```python
from build123d import *

# Parameters (mm, degrees)
SKETCH1_W                 = 100
SKETCH1_H                 = 100
BOSS_EXTRUDE1_DEPTH       = 52
SKETCH2_W                 = 95.5
SKETCH2_H                 = 95.5
BOSS_EXTRUDE2_DEPTH       = 2.5
SKETCH3_W                 = 96
SKETCH3_H                 = 96
CUT_EXTRUDE1_DEPTH        = 13
SKETCH4_R                 = 7.5
CUT_EXTRUDE2_DEPTH        = 37.5
LPATTERN1_COUNT           = 5
LPATTERN1_PITCH           = 17
LPATTERN1_COUNT_DIR2      = 3
LPATTERN1_PITCH_DIR2      = 30
SKETCH_PATTERN1_START     = 17
SKETCH_PATTERN1_OUTLINE_R = 7.5
SKETCH_PATTERN1_DEPTH     = 37.5
FILLET1_R                 = 5
FILLET2_R                 = 2


# Read off the part's stored shape, not the designer's step: Sketch-Pattern1
with BuildPart() as part:
    # Sketch1 → Boss-Extrude1 (new body)
    with BuildSketch(Plane.XY):
        Rectangle(SKETCH1_W, SKETCH1_H)
    extrude(amount=BOSS_EXTRUDE1_DEPTH)

    # Sketch2 → Boss-Extrude2 (add)
    with BuildSketch(Plane.XY.offset(52)):
        Rectangle(SKETCH2_W, SKETCH2_H)
    extrude(amount=BOSS_EXTRUDE2_DEPTH)

    # Sketch3 → Cut-Extrude1 (cut)
    with BuildSketch(Plane(origin=(0, 0, 0), x_dir=(-1, 0, 0), z_dir=(0, 0, -1))):
        Rectangle(SKETCH3_W, SKETCH3_H)
    extrude(amount=-CUT_EXTRUDE1_DEPTH, mode=Mode.SUBTRACT)

    # Sketch4 → Cut-Extrude2 (cut)
    with BuildSketch(Plane.XY.offset(54.5)):
        with Locations((38.75, 38.75)):
            Circle(SKETCH4_R)
    cut_extrude2 = extrude(amount=-CUT_EXTRUDE2_DEPTH, mode=Mode.SUBTRACT)

    # LPattern1: Cut-Extrude2 5 × 3
    with Locations(*[(-j * LPATTERN1_PITCH_DIR2, -i * LPATTERN1_PITCH, 0) for i in range(LPATTERN1_COUNT) for j in range(LPATTERN1_COUNT_DIR2) if (i, j) != (0, 0)]):
        add(cut_extrude2, mode=Mode.SUBTRACT)

    # Sketch-Pattern1 outline → Sketch-Pattern1 (cut)
    with BuildSketch(Plane.XY.offset(SKETCH_PATTERN1_START)):
        with Locations((23.75, 30.5)):
            Circle(SKETCH_PATTERN1_OUTLINE_R)
        with Locations((-36.25, 13.5)):
            Circle(SKETCH_PATTERN1_OUTLINE_R)
        with Locations((23.75, -3.5)):
            Circle(SKETCH_PATTERN1_OUTLINE_R)
        with Locations((-6.25, -3.5)):
            Circle(SKETCH_PATTERN1_OUTLINE_R)
        with Locations((-36.25, -3.5)):
            Circle(SKETCH_PATTERN1_OUTLINE_R)
        with Locations((-6.25, 13.5)):
            Circle(SKETCH_PATTERN1_OUTLINE_R)
        with Locations((23.75, 13.5)):
            Circle(SKETCH_PATTERN1_OUTLINE_R)
        with Locations((-36.25, 30.5)):
            Circle(SKETCH_PATTERN1_OUTLINE_R)
        with Locations((-6.25, 30.5)):
            Circle(SKETCH_PATTERN1_OUTLINE_R)
        with Locations((-36.25, -37.5)):
            Circle(SKETCH_PATTERN1_OUTLINE_R)
        with Locations((-6.25, -37.5)):
            Circle(SKETCH_PATTERN1_OUTLINE_R)
        with Locations((23.75, -20.5)):
            Circle(SKETCH_PATTERN1_OUTLINE_R)
        with Locations((-6.25, -20.5)):
            Circle(SKETCH_PATTERN1_OUTLINE_R)
        with Locations((-36.25, -20.5)):
            Circle(SKETCH_PATTERN1_OUTLINE_R)
        with Locations((23.75, -37.5)):
            Circle(SKETCH_PATTERN1_OUTLINE_R)
    extrude(amount=SKETCH_PATTERN1_DEPTH, mode=Mode.SUBTRACT)

    # Fillet1
    fillet1_edges = [part.edges().sort_by_distance(p)[0] for p in [
        (47.75, 47.75, 53.25),
        (-47.75, 47.75, 53.25),
        (-47.75, -47.75, 53.25),
        (47.75, -47.75, 53.25),
        (-48, -48, 6.5),
        (48, -48, 6.5),
        (48, 48, 6.5),
        (-48, 48, 6.5),
        (-50, 50, 26),
        (50, 50, 26),
        (50, -50, 26),
        (-50, -50, 26),
    ]]
    fillet(fillet1_edges, radius=FILLET1_R)

    # Fillet2
    fillet2_edges = [part.edges().sort_by_distance(p)[0] for p in [
        (0, -48, 13),
        (48, 0, 13),
        (-48, 0, 13),
        (0, 48, 13),
        (-46.535533906, 46.535533906, 13),
        (-46.535533906, -46.535533906, 13),
        (46.535533906, 46.535533906, 13),
        (46.535533906, -46.535533906, 13),
    ]]
    fillet(fillet2_edges, radius=FILLET2_R)


solid = part.part
```
Build history of the part. All positions in model axes, mm. A direction names the side the tool comes from. Coordinates: 2 decimals unless noted, no trailing zeros. Order: outer loops, then holes, each group sorted by start corner. A loop starts at its lowest first (then second) coordinate and runs counter-clockwise, first axis right, second up. Notation, with made-up numbers: (53.25, 35.5) -> (91.25, 35.5) arc R11 ccw to (91.25, 53.5) -> close; hole circle Ø11 at (13, -36.5). An arc over 180 degrees is marked (long way). Answer in a Markdown table with one row per item. Add a question column.
Q1. Drop flat-ended pins along their axis: pin 1 (12 mm diameter, centred on x = -16.5, y = -13.5, fed in from -Z); pin 2 (12 mm diameter, centred on x = -36.25, y = 30.5, fed in from +Z); pin 3 (0.8 mm diameter, centred on y = 5, z = 53, fed in from +X). Give the stop position or say it passes through.
Q2. Mould opens along X. For faces 4 (the face through (50, -1, 26)), 5 (the face through (1, 1, 13)), 6 (the face through (-47.75, -1, 53)) say: +X half, -X half, draft (parallel to the pull), parting line (faces both ways), or undercut.
Q3. Wall check: line 1 along Y through (x, z) = (23.75, 37); line 2 along X through (y, z) = (-21, 33.5); line 3 along X through (y, z) = (-12, 31). Give the ranges that are in metal, low to high. Write a range as [from, to].
Q4. Which spindle directions (+Z, -Z, +X, -X, +Y, -Y) get a long thin tool onto all of the face, cutting with end or side? Do faces 1 (the face through (9, 22, 17)), 2 (the face through (-46.25, -46.32, 53.27)), 3 (the face through (-48, -1, 5)). Say none if no direction does.
Q5. Band-saw the part on C-C, the plane z = 19. Give the number of separate pieces and of enclosed holes in the cut face, then the cut area to 3 significant figures.
Q6. Band-saw the part on A-A, the plane z = 5. List the corners of the cut face in (x, y), then the cut area to 3 significant figures.
Answers follow:
| question | item | result |
|---|---|---|
| 1 | pin 1 | z = 13 |
| 1 | pin 2 | z = 17 |
| 1 | pin 3 | x = 47.75 |
| 2 | face 4 | +X half |
| 2 | face 5 | undercut |
| 2 | face 6 | -X half |
| 3 | line 1 | [-50, -45], [-30, -28], [-13, -11], [4, 6], [21, 23], [38, 50] |
| 3 | line 2 | [-50, -43.73], [-28.77, -13.73], [1.23, 16.27], [31.23, 50] |
| 3 | line 3 | [-50, -28.75], [-13.75, 1.25], [16.25, 31.25], [46.25, 50] |
| 4 | face 1 | +Z |
| 4 | face 2 | +Z, -X, -Y |
| 4 | face 3 | -Z |
| 5 | separate pieces | 1 |
| 5 | enclosed holes | 30 |
| 5 | area | 4,680 mm^2 |
| 6 | outline | (-50, -45) arc R5 ccw to (-45, -50) -> (45, -50) arc R5 ccw to (50, -45) -> (50, 45) arc R5 ccw to (45, 50) -> (-45, 50) arc R5 ccw to (-50, 45) -> close; hole (-48, -43) arc R5 ccw to (-43, -48) -> (43, -48) arc R5 ccw to (48, -43) -> (48, 43) arc R5 ccw to (43, 48) -> (-43, 48) arc R5 ccw to (-48, 43) -> close |
| 6 | area | 784 mm^2 |
